Source: CAD feature listing. Evaluate the final solid. Frame: model axes, mm. A direction names the side the tool comes from. Coordinates: 2 decimals unless noted, no trailing zeros. Loops run counter-clockwise (first coordinate to the right, second up) from the corner with the lowest first, then second, coordinate; pieces in that order, holes last. Notation, with made-up numbers: (-0.75, 84.5) -> (18.25, 84.5) arc R15 cw to (18.25, 109.5) -> close; hole circle Ø2 at (-9.75, -22.5). An arc over 180 degrees is marked (long way). One line per question, with ' | ' between items. Start each with the question number.
```python
from build123d import *

# Parameters (mm, degrees)
BOSS_EXTRUDE1_DEPTH = 2.2
SKETCH2_R           = 1.5
BOSS_EXTRUDE2_DEPTH = 20
CHAMFER1_SIZE       = 0.3


with BuildPart() as part:
    # Sketch1 → Boss-Extrude1 (new body)
    with BuildSketch(Plane.XY):
        Polygon((2.592758174, -1.87552794), (2.920633928, 1.307630474), (0.327875755, 3.183158414), (-2.592758174, 1.87552794), (-2.920633928, -1.307630474), (-0.327875755, -3.183158414), align=None)
    extrude(amount=BOSS_EXTRUDE1_DEPTH)

    # Sketch2 → Boss-Extrude2 (add)
    with BuildSketch(Plane(origin=(0, 0, 0), x_dir=(-1, 0, 0), z_dir=(0, 0, -1))):
        with Locations(Location((0, 0, 0), (0, 0, 180))):
            Circle(SKETCH2_R)
    extrude(amount=BOSS_EXTRUDE2_DEPTH)

    # Chamfer1
    chamfer1_edges = [part.edges().sort_by_distance(p)[0] for p in [
        (-1.5, 0, -20),
    ]]
    chamfer(chamfer1_edges, length=CHAMFER1_SIZE)


solid = part.part
```
(1) Cut plane D-D, the plane x = -2.3. Return the cut outline in (y, z).
(2) Cut plane C-C, the plane x = 0. Return the cut outline in (y, z), and give its area (3 significant figures).
(3) Ray query, L1, parallel to Z at x = -2.4, y = 1.75; L2, parallel to Y at x = 1.3, z = -8; L3, parallel to Z at x = 1.3, y = 0.5. Return the intervals inside material, ascending.
(4) Cut plane B-B, the plane z = -4.75. Return the cut outline in (x, y), and give its area (3 significant figures).
(5) Access query for faces 1 (the flat face through (-0.7, 1.5, 0)), 2 (the flat face through (0, 0, -20)). Directions: +Z, -Z, +X, -X, +Y, -Y. A direction counts if a zero-diameter tool reaches every point of the face in a straight line with its end or side. Return the directions, or none.
(6) Contact query for a flat-ended pin moving along its axis: pin 1 Ø2 at (x, z) = (-2, -13) entering from +Y. Output: stop coordinate, or through.
(7) Cut plane A-A, the plane y = 0. Return the cut outline in (x, z), and give its area (3 significant figures).
Here are the results:
1) outline: (-1.76, 0) -> (2.01, 0) -> (2.01, 2.2) -> (-1.76, 2.2) -> close
2) outline: (-3.04, 0) -> (-1.5, 0) -> (-1.5, -19.7) -> (-1.2, -20) -> (1.2, -20) -> (1.5, -19.7) -> (1.5, 0) -> (3.04, 0) -> (3.04, 2.2) -> (-3.04, 2.2) -> close | area: 73.3 mm2
3) L1: z = 0 to 2.2 | L2: y = -0.75 to 0.75 | L3: z = -19.81 to 2.2
4) outline: circle Ø3 at (0, 0) | area: 7.07 mm2
5) face 1: -Z | face 2: -Z, +X, -X, +Y, -Y
6) pin 1: stops at y = 1.12
7) outline: (-2.79, 0) -> (-1.5, 0) -> (-1.5, -19.7) -> (-1.2, -20) -> (1.2, -20) -> (1.5, -19.7) -> (1.5, 0) -> (2.79, 0) -> (2.79, 2.2) -> (-2.79, 2.2) -> close | area: 72.2 mm2
